```python
from build123d import *

# Parameters (mm, degrees)
SKETCH_1_R      = 1.15
SKETCH_1_R_2    = 6.3
EXTRUDE_1_DEPTH = 2
SKETCH_2_R      = 12
SKETCH_2_R_2    = 10.5
EXTRUDE_2_DEPTH = 1.4
FILLET_1_R      = 7


with BuildPart() as part:
    # Эскиз1 → Бобышка-Вытянуть1 (new body)
    with BuildSketch(Plane(origin=(0, 0, 0), x_dir=(1, 0, 0), z_dir=(0, 1, 0))):
        with BuildLine():
            ThreePointArc((-5.15088911, 13.27576519), (-12.33220175, 7.12), (-14.072594464, -2.177081774))
            ThreePointArc((-14.072594464, -2.177081774), (-14.376715993, -4.021792929), (-15.714174027, -5.328183054))
            ThreePointArc((-15.714174027, -5.328183054), (-17.095341471, -9.87), (-12.471428894, -10.94478238))
            ThreePointArc((-12.471428894, -10.94478238), (-10.671332842, -10.439704809), (-8.921705354, -11.098683416))
            ThreePointArc((-8.921705354, -11.098683416), (0, -14.24), (8.921705354, -11.098683416))
            ThreePointArc((8.921705354, -11.098683416), (10.671332842, -10.439704809), (12.471428894, -10.94478238))
            ThreePointArc((12.471428894, -10.94478238), (17.095341471, -9.87), (15.714174027, -5.328183054))
            ThreePointArc((15.714174027, -5.328183054), (14.376715993, -4.021792929), (14.072594464, -2.177081774))
            ThreePointArc((14.072594464, -2.177081774), (12.33220175, 7.12), (5.15088911, 13.27576519))
            ThreePointArc((5.15088911, 13.27576519), (3.705383152, 14.461497738), (3.242745133, 16.272965434))
            ThreePointArc((3.242745133, 16.272965434), (0, 19.74), (-3.242745133, 16.272965434))
            ThreePointArc((-3.242745133, 16.272965434), (-3.705383152, 14.461497738), (-5.15088911, 13.27576519))
        make_face()
        with Locations(Location((0, 16.49, 0), (0, 0, 270))):
            Circle(SKETCH_1_R, mode=Mode.SUBTRACT)
        with Locations(Location((0, 0, 0), (0, 0, 270))):
            Circle(SKETCH_1_R_2, mode=Mode.SUBTRACT)
        with Locations(Location((14.280758908, -8.245, 0), (0, 0, 270))):
            Circle(SKETCH_1_R, mode=Mode.SUBTRACT)
        with Locations(Location((-14.280758908, -8.245, 0), (0, 0, 270))):
            Circle(SKETCH_1_R, mode=Mode.SUBTRACT)
    extrude(amount=EXTRUDE_1_DEPTH)

    # Эскиз2 → Бобышка-Вытянуть2 (add)
    with BuildSketch(Plane(origin=(0, 2, 0), x_dir=(1, 0, 0), z_dir=(0, 1, 0))):
        with Locations(Location((0, 0, 0), (0, 0, 270))):
            Circle(SKETCH_2_R)
        with Locations(Location((0, 0, 0), (0, 0, 270))):
            Circle(SKETCH_2_R_2, mode=Mode.SUBTRACT)
    extrude(amount=EXTRUDE_2_DEPTH)

    # Скругление1
    # the kernel refuses this fillet: 7 mm, written as the material it adds along each edge
    with BuildSketch(Plane(origin=(0, 2, 0), x_dir=(0, 0, 1), z_dir=(-1, 0, 0))) as fillet_1_piece_1:
        with BuildLine():
            CenterArc((6.3, 7), FILLET_1_R, 270, 36.869897646)
            Line((10.5, 1.4), (10.5, 0))
            Line((10.5, 0), (6.3, 0))
        make_face()
    revolve(axis=Axis((0, 2, 0), (0, 1, 0)))


solid = part.part
```
Source: CAD feature listing. Evaluate the final solid. Frame: model axes, mm. A direction names the side the tool comes from. Give positions to 0.01 mm unless a question says otherwise; leave off trailing zeros. Loops run counter-clockwise (first coordinate to the right, second up) from the corner with the lowest first, then second, coordinate; pieces in that order, holes last. Notation, with made-up numbers: (-1.5, -16.75) - (50.5, -16.75) arc R22 cw to (50.5, 18.25) - close; hole circle Ø6 at (51, 27.5). An arc over 180 degrees is marked (long way). Use CSV: the item, a comma, the result in double quotes.
1) Cut plane C-C (x = 11). Output: boundary loops of the cut face in (y, z), and give its area (3 significant figures).
Worked out:
outline,"(0, -9.04) - (2, -9.04) - (2, -4.8) - (3.4, -4.8) - (3.4, 4.8) - (2, 4.8) - (2, 10.44) - (0, 10.44) - close"
area,"52.4 mm^2"
2) Cut plane A-A (y = 0.65). Output: boundary loops of the cut face in (x, z) (3 decimals), and give its area (3 significant figures).
Worked out:
outline,"(-15.714, 5.328) arc R3 cw to (-14.073, 2.177) arc R14.24 ccw to (-5.151, -13.276) arc R3 cw to (-3.243, -16.273) arc R3.25 ccw (long way) to (3.243, -16.273) arc R3 cw to (5.151, -13.276) arc R14.24 ccw to (14.073, 2.177) arc R3 cw to (15.714, 5.328) arc R3.25 ccw (long way) to (12.471, 10.945) arc R3 cw to (8.922, 11.099) arc R14.24 ccw to (-8.922, 11.099) arc R3 cw to (-12.471, 10.945) arc R3.25 ccw (long way) to start; hole circle Ø2.3 at (-14.281, 8.245); hole circle Ø12.6 at (0, 0); hole circle Ø2.3 at (0, -16.49); hole circle Ø2.3 at (14.281, 8.245)"
area,"601 mm^2"
3) Pin query (flat end, axial travel): P1, Ø2, axis at y = 2.5, z = -3.5, coming from the -X side; P2, Ø17, axis at x = -3.5, z = -8, coming from the +Y side; P3, Ø2, axis at x = -5, y = 0.5, coming from the +Z side; P4, Ø1, axis at y = 1.5, z = -8, coming from the -X side. Return the tip coordinate at first contact, or that it passes through.
Worked out:
P1,"stops at x = -13.99"
P2,"stops at y = 3.4"
P3,"stops at z = 13.67"
P4,"stops at x = -12.1"
4) Mould query, pull axis X, two halves, no side actions, for faces 3 (the cylindrical face through (14.39, 0.99, 4.05)), 4 (the flat face through (-7, 2, -10)), 5 (the cylindrical face through (10.64, 0.99, 10.44)), 6 (the cylindrical face through (17.06, 0.99, 9.93)). Classes: +X half, -X half, draft (parallel to the pull), parting line (faces both ways), or undercut.
Worked out:
face 3,"+X half"
face 4,"draft"
face 5,"undercut"
face 6,"undercut"
5) Line query: line 1 (X direction, y = 1.4, z = -16.49); line 2 (Y direction, x = 13, z = 1.5); line 3 (X direction, y = 1.2, z = -3). Output: solid intervals per line, ascending.
Worked out:
line 1,"x = -3.25 to -1.15, 1.15 to 3.25"
line 2,"y = 0 to 2"
line 3,"x = -13.92 to -5.54, 5.54 to 13.92"
6) Cut plane B-B (x = 0). Count the separate pieces of the cut face and the enclosed holes in it, and give its area (3 significant figures).
Worked out:
separate pieces,"3"
enclosed holes,"0"
area,"46.1 mm^2"
7) Set-up query: faces 1 (the cylindrical face through (3.604, 2.69, 11.446)), 2 (the cylindrical face through (-17.13, 0.99, 9.81)). Return all of +Z, -Z, +X, -X, +Y, -Y with unobstructed straight access to the full face (end or side cutting, diameter ignored); none if empty.
Worked out:
face 1,"+Y"
face 2,"+Y, -Y"
